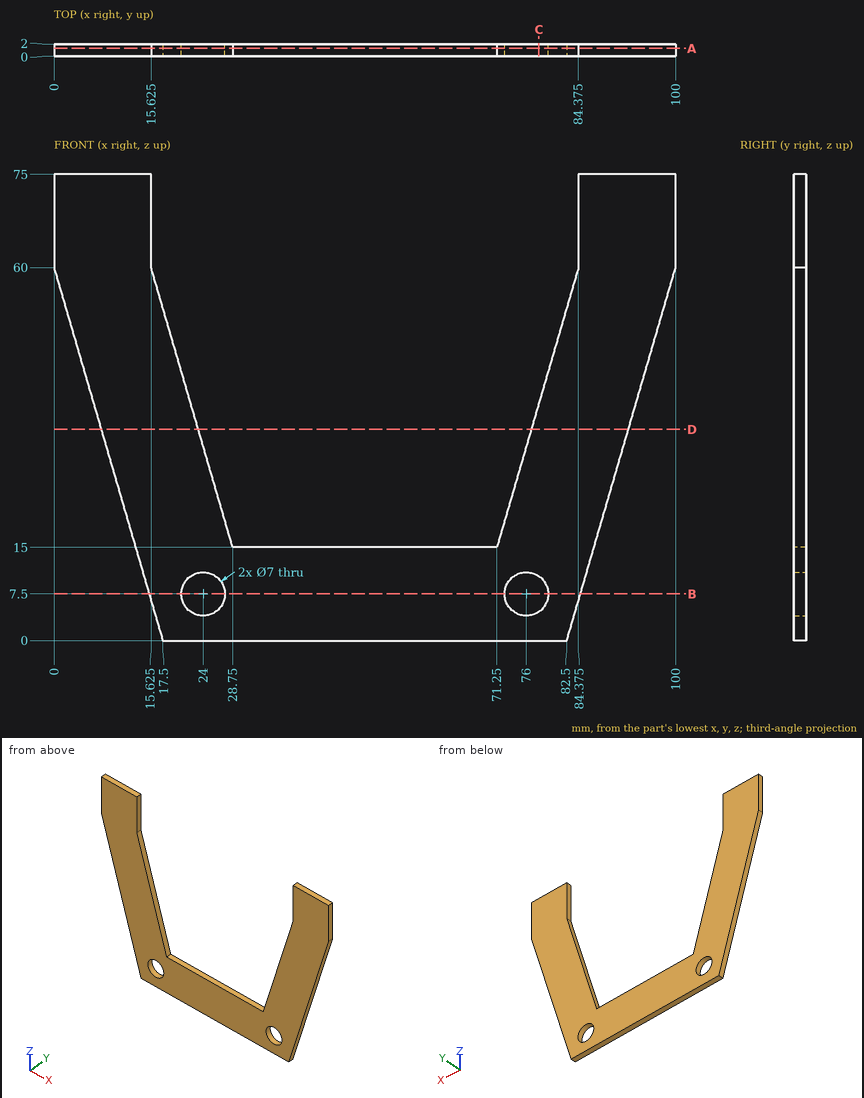
Study the drawing (mm; zero at the part's minimum x, y, z) and answer. Coordinates: 2 decimals unless noted, no trailing zeros. Order: outer loops, then holes, each group sorted by start corner. A loop starts at its lowest first (then second) coordinate and runs counter-clockwise, first axis right, second up. Notation, with made-up numbers: (29, -16) -> (69, -16) arc R15 ccw to (69, 4) -> close; hole circle Ø1 at (42.5, -33). An arc over 180 degrees is marked (long way). Answer in a Markdown table with one row per item. Add a question column.
Item 1: Find section B-B (z = 7.5). Write down the section's boundary in (x, y), then the cut area to 3 significant figures.
Item 2: Find the intervals of material crossed by L1, parallel to X at y = 0.1, z = 67 (3 decimals); L2, parallel to X at y = 1.15, z = 30 (3 decimals); L3, parallel to Z at x = 65, y = 1.5, in increasing order. Write a range as from..to.
Item 3: Find section C-C (x = 78). Write down the section's boundary in (y, z), then the cut area to 3 significant figures.
Item 4: Find section A-A (y = 1.3). Write down the section's boundary in (x, z) (3 decimals), then the cut area to 3 significant figures.
Item 5: Find section D-D (z = 34). Write down the section's boundary in (x, y), then the cut area to 3 significant figures.
Result set:
| question | item | result |
|---|---|---|
| 1 | outline | (15.31, 0) -> (20.5, 0) -> (20.5, 2) -> (15.31, 2) -> close; (27.5, 0) -> (72.5, 0) -> (72.5, 2) -> (27.5, 2) -> close; (79.5, 0) -> (84.69, 0) -> (84.69, 2) -> (79.5, 2) -> close |
| 1 | area | 111 mm² |
| 2 | L1 | x = 0..15.625, 84.375..100 |
| 2 | L2 | x = 8.75..24.375, 75.625..91.25 |
| 2 | L3 | z = 0..15 |
| 3 | outline | (0, 0) -> (2, 0) -> (2, 4.63) -> (0, 4.63) -> close; (0, 10.37) -> (2, 10.37) -> (2, 38.14) -> (0, 38.14) -> close |
| 3 | area | 64.8 mm² |
| 4 | outline | (0, 60) -> (17.5, 0) -> (82.5, 0) -> (100, 60) -> (100, 75) -> (84.375, 75) -> (84.375, 60) -> (71.25, 15) -> (28.75, 15) -> (15.625, 60) -> (15.625, 75) -> (0, 75) -> close; hole circle Ø7 at (24, 7.5); hole circle Ø7 at (76, 7.5) |
| 4 | area | 2,840 mm² |
| 5 | outline | (7.58, 0) -> (23.21, 0) -> (23.21, 2) -> (7.58, 2) -> close; (76.79, 0) -> (92.42, 0) -> (92.42, 2) -> (76.79, 2) -> close |
| 5 | area | 62.5 mm² |
